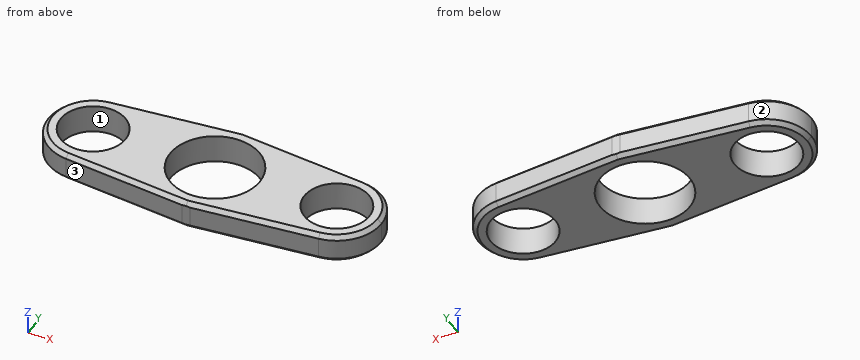
```python
from build123d import *

# Parameters (mm, degrees)
F0_W         = 82
F0_H         = 28
F0_R         = 8
F0_R_2       = 11.05
F1_DEPTH     = 7
F2_SIZE2     = 4
F2_SIZE      = 40
F2_2_SIZE2   = 4
F2_2_SIZE    = 40
F3_R         = 11
F4_T1_DEPTH  = 43.1030542411
F4_T3_DEPTH  = 43.1030542411
F4_T5_DEPTH  = 43.1030542411
F4_T7_DEPTH  = 43.1030542411
F4_T9_DEPTH  = 0.0902736335
F4_T12_ANGLE = 84.2894068625
F4_T14_ANGLE = 84.2894068625
F4_T16_ANGLE = 84.2894068625
F4_T18_ANGLE = 84.2894068625
F4_T20_ANGLE = 84.2894068625
F4_T22_ANGLE = 84.2894068625
F4_T24_ANGLE = 84.2894068625
F4_T26_ANGLE = 84.2894068625


# Not quite as in the source:
# - a fillet or chamfer that OpenCascade refuses, or shapes differently, is made with other operations: its cross-section is extruded or revolved along the edge and cut away or added


with BuildPart() as f1:
    # F0 (on Top) → F1 (new body)
    with BuildSketch(Plane.XY):
        Rectangle(F0_W, F0_H)
        with Locations((-30, 0)):
            Circle(F0_R, mode=Mode.SUBTRACT)
        Circle(F0_R_2, mode=Mode.SUBTRACT)
        with Locations((30, 0)):
            Circle(F0_R, mode=Mode.SUBTRACT)
    extrude(amount=F1_DEPTH)

    # F2
    f2_edges = [f1.edges().sort_by_distance(p)[0] for p in [
        (-41, -14, 3.5),
        (41, -14, 3.5),
    ]]
    f2_side = f1.faces().sort_by_distance((0, -14, 3.5))[0]
    chamfer(f2_edges, length=F2_SIZE, length2=F2_SIZE2, reference=f2_side)

    # F2#2
    f2_2_edges = [f1.edges().sort_by_distance(p)[0] for p in [
        (41, 14, 3.5),
        (-41, 14, 3.5),
    ]]
    f2_2_side = f1.faces().sort_by_distance((0, 14, 3.5))[0]
    chamfer(f2_2_edges, length=F2_2_SIZE, length2=F2_2_SIZE2, reference=f2_2_side)

    # F3
    f3_edges = [f1.edges().sort_by_distance(p)[0] for p in [
        (-41, 10, 3.5),
        (-41, -10, 3.5),
        (41, 10, 3.5),
        (41, -10, 3.5),
    ]]
    fillet(f3_edges, radius=F3_R)

    # F4: chamfer of 1 on 20 edges, made by hand

    # F4_s2 → F4_t1 (cut)
    with BuildSketch(Plane(origin=(13.1906406762, -1.3190640676, 0), x_dir=(0, 0, 1), z_dir=(-0.9950371902, 0.099503719, 0))):
        Polygon((7, -13.030024382), (6, -14.030024382), (7, -14.030024382), align=None)
        Polygon((0, -13.030024382), (1, -14.030024382), (0, -14.030024382), align=None)
    extrude(amount=F4_T1_DEPTH, mode=Mode.SUBTRACT)

    # F4_s4 → F4_t3 (cut)
    with BuildSketch(Plane(origin=(-13.1906406762, -1.3190640676, 0), x_dir=(0, 0, 1), z_dir=(0.9950371902, 0.099503719, 0))):
        Polygon((7, 13.030024382), (6, 14.030024382), (7, 14.030024382), align=None)
        Polygon((0, 13.030024382), (1, 14.030024382), (0, 14.030024382), align=None)
    extrude(amount=F4_T3_DEPTH, mode=Mode.SUBTRACT)

    # F4_s6 → F4_t5 (cut)
    with BuildSketch(Plane(origin=(-13.1906406762, 1.3190640676, 0), x_dir=(0, 0, 1), z_dir=(0.9950371902, -0.099503719, 0))):
        Polygon((7, -13.030024382), (6, -14.030024382), (7, -14.030024382), align=None)
        Polygon((0, -13.030024382), (1, -14.030024382), (0, -14.030024382), align=None)
    extrude(amount=F4_T5_DEPTH, mode=Mode.SUBTRACT)

    # F4_s8 → F4_t7 (cut)
    with BuildSketch(Plane(origin=(13.1906406762, 1.3190640676, 0), x_dir=(0, 0, 1), z_dir=(-0.9950371902, -0.099503719, 0))):
        Polygon((7, 13.030024382), (6, 14.030024382), (7, 14.030024382), align=None)
        Polygon((0, 13.030024382), (1, 14.030024382), (0, 14.030024382), align=None)
    extrude(amount=F4_T7_DEPTH, mode=Mode.SUBTRACT)

    # F4_s10 → F4_t9 (cut)
    with BuildSketch(Plane.XZ.offset(-0.0451368168)):
        Polygon((41, 1), (40, 0), (41, 0), align=None)
        Polygon((41, 6), (40, 7), (41, 7), align=None)
        Polygon((-40, 0), (-41, 1), (-41, 0), align=None)
        Polygon((-40, 7), (-41, 6), (-41, 7), align=None)
    extrude(amount=F4_T9_DEPTH, mode=Mode.SUBTRACT)

    # F4_s11 → F4_t12 (revolve, cut)
    with BuildSketch(Plane.XZ.offset(0.0451368168)):
        Polygon((40, 0), (41, 1), (41, 0), align=None)
    revolve(axis=Axis((30, -0.0451368168, 0), (0, 0, -1)), revolution_arc=F4_T12_ANGLE, mode=Mode.SUBTRACT)

    # F4_s13 → F4_t14 (revolve, cut)
    with BuildSketch(Plane.XZ.offset(-0.0451368168)):
        Polygon((40, 0), (41, 1), (41, 0), align=None)
    revolve(axis=Axis((30, 0.0451368168, 0), (0, 0, 1)), revolution_arc=F4_T14_ANGLE, mode=Mode.SUBTRACT)

    # F4_s15 → F4_t16 (revolve, cut)
    with BuildSketch(Plane(origin=(-29.6985013053, 2.9698501305, 0), x_dir=(0, 0, 1), z_dir=(0.9950371902, -0.099503719, 0))):
        Polygon((0, 13.030024382), (1, 14.030024382), (0, 14.030024382), align=None)
    revolve(axis=Axis((-30, -0.0451368168, 0), (0, 0, -1)), revolution_arc=F4_T16_ANGLE, mode=Mode.SUBTRACT)

    # F4_s17 → F4_t18 (revolve, cut)
    with BuildSketch(Plane(origin=(-29.6985013053, -2.9698501305, 0), x_dir=(0, 0, 1), z_dir=(0.9950371902, 0.099503719, 0))):
        Polygon((0, -13.030024382), (1, -14.030024382), (0, -14.030024382), align=None)
    revolve(axis=Axis((-30, 0.0451368168, 0), (0, 0, 1)), revolution_arc=F4_T18_ANGLE, mode=Mode.SUBTRACT)

    # F4_s19 → F4_t20 (revolve, cut)
    with BuildSketch(Plane.XZ.offset(0.0451368168)):
        Polygon((41, 6), (40, 7), (41, 7), align=None)
    revolve(axis=Axis((30, -0.0451368168, 7), (0, 0, -1)), revolution_arc=F4_T20_ANGLE, mode=Mode.SUBTRACT)

    # F4_s21 → F4_t22 (revolve, cut)
    with BuildSketch(Plane.XZ.offset(-0.0451368168)):
        Polygon((41, 6), (40, 7), (41, 7), align=None)
    revolve(axis=Axis((30, 0.0451368168, 7), (0, 0, 1)), revolution_arc=F4_T22_ANGLE, mode=Mode.SUBTRACT)

    # F4_s23 → F4_t24 (revolve, cut)
    with BuildSketch(Plane(origin=(-29.6985013053, 2.9698501305, 0), x_dir=(0, 0, 1), z_dir=(0.9950371902, -0.099503719, 0))):
        Polygon((7, 13.030024382), (6, 14.030024382), (7, 14.030024382), align=None)
    revolve(axis=Axis((-30, -0.0451368168, 7), (0, 0, -1)), revolution_arc=F4_T24_ANGLE, mode=Mode.SUBTRACT)

    # F4_s25 → F4_t26 (revolve, cut)
    with BuildSketch(Plane(origin=(-29.6985013053, -2.9698501305, 0), x_dir=(0, 0, 1), z_dir=(0.9950371902, 0.099503719, 0))):
        Polygon((7, -13.030024382), (6, -14.030024382), (7, -14.030024382), align=None)
    revolve(axis=Axis((-30, 0.0451368168, 7), (0, 0, 1)), revolution_arc=F4_T26_ANGLE, mode=Mode.SUBTRACT)


solid = f1.part
```
Work out the finished part from the listing and answer in its coordinate system (mm). Face numbers are marked on the shaded views. Give positions to 0.01 mm unless a question says otherwise; leave off trailing zeros. Write each loop counter-clockwise with the first axis right and the second up, starting at its lowest first coordinate (ties: lowest second). Pieces come first, ordered by that corner, then holes. Notation, with made-up numbers: (41.25, 8.5) - (59.25, 8.5) arc R23 cw to (59.25, 31.5) - close; hole circle Ø3 at (63.25, -33). An arc over 180 degrees is marked (long way). Use one line per item in the form item = value.
1. A cutting plane is placed at B-B (x = 28). Write down the section's boundary in (y, z).
Filled in:
outline = (-11.3, 1) - (-10.3, 0) - (-7.75, 0) - (-7.75, 7) - (-10.3, 7) - (-11.3, 6) - close; (7.75, 0) - (10.3, 0) - (11.3, 1) - (11.3, 6) - (10.3, 7) - (7.75, 7) - close
2. A cutting plane is placed at D-D (x = -8). Write down the section's boundary in (y, z).
Filled in:
outline = (-13.3, 1) - (-12.3, 0) - (-7.62, 0) - (-7.62, 7) - (-12.3, 7) - (-13.3, 6) - close; (7.62, 0) - (12.3, 0) - (13.3, 1) - (13.3, 6) - (12.3, 7) - (7.62, 7) - close
3. A cutting plane is placed at A-A (z = 2.5). Write down the section's boundary in (x, y), and give its area (3 significant figures).
Filled in:
outline = (-41, -0.05) arc R11 ccw to (-31.09, -10.99) - (-1, -14) - (1, -14) - (31.09, -10.99) arc R11 ccw to (41, -0.05) - (41, 0.05) arc R11 ccw to (31.09, 10.99) - (1, 14) - (-1, 14) - (-31.09, 10.99) arc R11 ccw to (-41, 0.05) - close; hole circle Ø16 at (-30, 0); hole circle Ø22.1 at (0, 0); hole circle Ø16 at (30, 0)
area = 1,110 mm^2
4. Consider L1, parallel to X at y = 2, z = 4.75; L2, parallel to X at y = -3.5, z = 5.75; L3, parallel to Y at x = 30, z = 2.5. Determine where each line is inside the solid, lowest interval first.
Filled in:
L1 = -40.82 to -37.75, -22.25 to -10.87, 10.87 to 22.25, 37.75 to 40.82
L2 = -40.44 to -37.19, -22.81 to -10.48, 10.48 to 22.81, 37.19 to 40.44
L3 = -11.1 to -8, 8 to 11.1
5. Determine the mould class of the marked faces 1, 2 and 3 for opening direction Y: released by +Y, released by -Y, zero draft, split by the parting line, or undercut.
Filled in:
face_1 = undercut
face_2 = released by +Y
face_3 = released by -Y
6. Each of these flat-tipped pins is pushed along its axis until it touches: pin 1 Ø1.5 at (x, z) = (21.5, 6) entering from +Y (3 decimals); pin 2 Ø13 at (x, y) = (30, 0) entering from +Z. Where does it stop, or does it pass through?
Filled in:
pin_1 = 12.025
pin_2 = through
7. A cutting plane is placed at C-C (y = -4.25). State how many separate pieces and enclosed holes the cut face has, and give its area (3 significant figures).
Filled in:
separate_pieces = 4
enclosed_holes = 0
area = 228 mm^2
